```python
from build123d import *

# Parameters (mm, degrees)
BOSS_EXTRUDE1_DEPTH = 50.8
SKETCH3_R           = 1.27
CUT_EXTRUDE2_DEPTH  = 50.8
CUT_EXTRUDE1_DEPTH  = 50.8
CUT_EXTRUDE6_DEPTH  = 50.8
BOSS_EXTRUDE3_DEPTH = 20.32
SKETCH4_W           = 10.16
SKETCH4_H           = 15.24
CUT_EXTRUDE3_DEPTH  = 50.8
SKETCH5_R           = 2.54
CUT_EXTRUDE5_DEPTH  = 50.8
SKETCH8_R           = 2.54
BOSS_EXTRUDE2_DEPTH = 2.54
LPATTERN1_COUNT     = 2
LPATTERN1_PITCH     = 12.7
CUT_EXTRUDE7_DEPTH  = 20.32
SKETCH12_W          = 5.08
SKETCH12_H          = 19.941398178
CUT_EXTRUDE8_DEPTH  = 21.59
CUT_EXTRUDE9_DEPTH  = 5.08
LPATTERN2_COUNT     = 2
LPATTERN2_PITCH     = 15.24
CUT_EXTRUDE10_DEPTH = 40.767
BOSS_EXTRUDE4_START = 2.54
SKETCH16_R          = 7.638081415
BOSS_EXTRUDE4_DEPTH = 2.54
SKETCH17_R          = 2.54
CUT_EXTRUDE11_DEPTH = 2.54
SKETCH23_W          = 3.776239755
SKETCH23_H          = 7.410355269
CUT_EXTRUDE16_DEPTH = 2.54
CUT_EXTRUDE17_DEPTH = 9.906
SKETCH25_R          = 1.7526
CUT_EXTRUDE18_DEPTH = 20.828
SKETCH26_R          = 2.921
CUT_EXTRUDE19_DEPTH = 2.54


with BuildPart() as part:
    # Sketch1 → Boss-Extrude1 (new body)
    with BuildSketch(Plane(origin=(0, 0, 0), x_dir=(1, 0, 0), z_dir=(0, 1, 0))):
        with BuildLine():
            Line((-20.32, 27.095319289), (-20.32, 11.855319289))
            ThreePointArc((-20.32, 11.855319289), (-19.204076836, 9.161242453), (-16.51, 8.045319289))
            Line((-16.51, 8.045319289), (-3.81, 8.045319289))
            ThreePointArc((-3.81, 8.045319289), (-1.115923164, 9.161242453), (0, 11.855319289))
            Line((0, 11.855319289), (0, 27.095319289))
            ThreePointArc((0, 27.095319289), (-1.115923164, 29.789396126), (-3.81, 30.905319289))
            Line((-3.81, 30.905319289), (-16.51, 30.905319289))
            ThreePointArc((-16.51, 30.905319289), (-19.204076836, 29.789396126), (-20.32, 27.095319289))
        make_face()
    extrude(amount=BOSS_EXTRUDE1_DEPTH)

    # Sketch3 → Cut-Extrude2 (cut)
    with BuildSketch(Plane(origin=(0, 50.8, 0), x_dir=(1, 0, 0), z_dir=(0, 1, 0))):
        with Locations(Location((-10.16, 10.585319289, 0), (0, 0, 270))):
            Circle(SKETCH3_R)
        with Locations(Location((-10.16, 28.365319289, 0), (0, 0, 270))):
            Circle(SKETCH3_R)
    extrude(amount=-CUT_EXTRUDE2_DEPTH, mode=Mode.SUBTRACT)

    # Sketch2 → Cut-Extrude1 (cut)
    with BuildSketch(Plane.ZY.offset(20.32)):
        with BuildLine():
            Line((-27.095319289, 7.62), (-30.905319289, 15.24))
            Line((-30.905319289, 15.24), (-30.905319289, -5.08))
            Line((-30.905319289, -5.08), (-8.045319289, -5.08))
            Line((-8.045319289, -5.08), (-8.045319289, 15.24))
            Line((-8.045319289, 15.24), (-11.855319289, 7.62))
            ThreePointArc((-11.855319289, 7.62), (-19.475319289, 0), (-27.095319289, 7.62))
        make_face()
        with BuildLine():
            Line((-11.821559044, 42.970355269), (-8.045319289, 35.56))
            Line((-8.045319289, 35.56), (-8.045319289, 55.88))
            Line((-8.045319289, 55.88), (-30.905319289, 55.88))
            Line((-30.905319289, 55.88), (-30.905319289, 35.56))
            Line((-30.905319289, 35.56), (-27.092422036, 42.951560486))
            ThreePointArc((-27.092422036, 42.951560486), (-19.46663852, 50.799994215), (-11.821559044, 42.970355269))
        make_face()
    extrude(amount=-CUT_EXTRUDE1_DEPTH, mode=Mode.SUBTRACT)

    # Sketch7 → Cut-Extrude6 (cut)
    with BuildSketch(Plane.XY.offset(-8.045319289)):
        Polygon((-15.24, 50.8), (-12.7, 50.8), (-12.7, 35.56), (-7.62, 35.56), (-7.62, 50.8), (-5.08, 50.8), (-5.08, 35.56), (0, 35.56), (0, 59.156438057), (-20.32, 59.156438057), (-20.32, 35.56), (-15.24, 35.56), align=None)
    extrude(amount=-CUT_EXTRUDE6_DEPTH, mode=Mode.SUBTRACT)

    # Sketch9 → Boss-Extrude3 (add)
    with BuildSketch(Plane.ZY.offset(20.32)):
        with BuildLine():
            Line((-19.475319289, 35.56), (-30.961107471, 35.56))
            Line((-30.961107471, 35.56), (-30.961107471, 45.935432902))
            ThreePointArc((-30.961107471, 45.935432902), (-30.291229548, 47.014503778), (-29.026975399, 46.892882091))
            Line((-29.026975399, 46.892882091), (-27.092843326, 42.985764183))
            ThreePointArc((-27.092843326, 42.985764183), (-24.794356941, 37.723605727), (-19.475319289, 35.56))
        make_face()
    extrude(amount=-BOSS_EXTRUDE3_DEPTH)

    # Sketch4 → Cut-Extrude3 (cut)
    with BuildSketch(Plane.XY.offset(-8.045319289)):
        with Locations((-10.16, 7.62)):
            Rectangle(SKETCH4_W, SKETCH4_H)
    extrude(amount=-CUT_EXTRUDE3_DEPTH, mode=Mode.SUBTRACT)

    # Sketch5 → Cut-Extrude5 (cut)
    with BuildSketch(Plane.ZY.offset(20.32)):
        with Locations((-19.475319289, 7.62)):
            Circle(SKETCH5_R)
    extrude(amount=-CUT_EXTRUDE5_DEPTH, mode=Mode.SUBTRACT)

    # Sketch8 → Boss-Extrude2 (add)
    with BuildSketch(Plane.ZY.offset(15.24)):
        with Locations(Location((-19.441559044, 43.179995622, 0), (0, 0, 180))):
            Circle(SKETCH8_R)
    boss_extrude2 = extrude(amount=BOSS_EXTRUDE2_DEPTH)

    # LPattern1: Boss-Extrude2 ×2
    with Locations(*[(i * LPATTERN1_PITCH, 0, 0) for i in range(1, LPATTERN1_COUNT)]):
        add(boss_extrude2)

    # Sketch10 → Cut-Extrude7 (cut)
    with BuildSketch(Plane.XZ.offset(-35.56)):
        with BuildLine():
            Line((-16.51, -30.905319289), (-3.81, -30.905319289))
            ThreePointArc((-3.81, -30.905319289), (-1.115923164, -29.789396126), (0, -27.095319289))
            Line((0, -27.095319289), (5.770912039, -37.258829719))
            Line((5.770912039, -37.258829719), (-26.797758959, -37.890739908))
            Line((-26.797758959, -37.890739908), (-20.32, -27.095319289))
            ThreePointArc((-20.32, -27.095319289), (-19.204076836, -29.789396126), (-16.51, -30.905319289))
        make_face()
    extrude(amount=-CUT_EXTRUDE7_DEPTH, mode=Mode.SUBTRACT)

    # Sketch12 → Cut-Extrude8 (cut)
    with BuildSketch(Plane.XY.offset(-8.045319289)):
        with Locations((-10.16, 45.530699089)):
            Rectangle(SKETCH12_W, SKETCH12_H)
    extrude(amount=-CUT_EXTRUDE8_DEPTH, mode=Mode.SUBTRACT)

    # Sketch13 → Cut-Extrude9 (cut)
    with BuildSketch(Plane.ZY.offset(20.32)):
        Polygon((-19.475319289, 35.56), (-8.045319289, 30.82545932), (-1.320705488, 30.82545932), (-1.320705488, 35.56), align=None)
    cut_extrude9 = extrude(amount=-CUT_EXTRUDE9_DEPTH, mode=Mode.SUBTRACT)

    # LPattern2: Cut-Extrude9 ×2
    with Locations(*[(i * LPATTERN2_PITCH, 0, 0) for i in range(1, LPATTERN2_COUNT)]):
        add(cut_extrude9, mode=Mode.SUBTRACT)

    # Sketch15 → Cut-Extrude10 (cut, symmetric)
    with BuildSketch(Plane(origin=(0, 35.56, 0), x_dir=(1, 0, 0), z_dir=(0, 1, 0))):
        with BuildLine():
            Line((-10.16, 25.825319289), (-10.16, 13.125319289))
            ThreePointArc((-10.16, 13.125319289), (-7.62, 10.585319289), (-10.16, 8.045319289))
            Line((-10.16, 8.045319289), (-39.973745678, -4.467023153))
            Line((-39.973745678, -4.467023153), (-44.095820535, 43.963158694))
            Line((-44.095820535, 43.963158694), (-10.16, 30.905319289))
            ThreePointArc((-10.16, 30.905319289), (-12.7, 28.365319289), (-10.16, 25.825319289))
        make_face()
    extrude(amount=CUT_EXTRUDE10_DEPTH, both=True, mode=Mode.SUBTRACT)

    # Sketch16 → Boss-Extrude4 (add)
    with BuildSketch(Plane.ZY.offset(7.62).offset(BOSS_EXTRUDE4_START)):
        with Locations((-19.457237874, 43.161918585)):
            Circle(SKETCH16_R)
    extrude(amount=-BOSS_EXTRUDE4_DEPTH)

    # Sketch17 → Cut-Extrude11 (cut)
    with BuildSketch(Plane.ZY.offset(10.16)):
        with Locations((-19.457237874, 43.161918585)):
            Circle(SKETCH17_R)
    extrude(amount=-CUT_EXTRUDE11_DEPTH, mode=Mode.SUBTRACT)

    # Sketch23 → Cut-Extrude16 (cut)
    with BuildSketch(Plane(origin=(-5.08, 0, 0), x_dir=(0, 0, -1), z_dir=(1, 0, 0))):
        with Locations((9.933439167, 39.265177635)):
            Rectangle(SKETCH23_W, SKETCH23_H)
    extrude(amount=-CUT_EXTRUDE16_DEPTH, mode=Mode.SUBTRACT)

    # Sketch24 → Cut-Extrude17 (cut)
    with BuildSketch(Plane(origin=(-5.08, 0, 0), x_dir=(0, 0, -1), z_dir=(1, 0, 0))):
        Polygon((8.045319289, 35.56), (11.821559044, 35.56), (11.821559044, 32.38965536), (8.045319289, 30.82545932), align=None)
    extrude(amount=-CUT_EXTRUDE17_DEPTH, mode=Mode.SUBTRACT)

    # Sketch25 → Cut-Extrude18 (cut)
    with BuildSketch(Plane.ZY.offset(10.16)):
        with Locations((-19.475319289, 22.86)):
            Circle(SKETCH25_R)
    extrude(amount=-CUT_EXTRUDE18_DEPTH, mode=Mode.SUBTRACT)

    # Sketch26 → Cut-Extrude19 (cut)
    with BuildSketch(Plane(origin=(0, 0, 0), x_dir=(0, 0, -1), z_dir=(1, 0, 0))):
        with Locations((19.475319289, 22.86)):
            Circle(SKETCH26_R)
    extrude(amount=-CUT_EXTRUDE19_DEPTH, mode=Mode.SUBTRACT)


solid = part.part
```
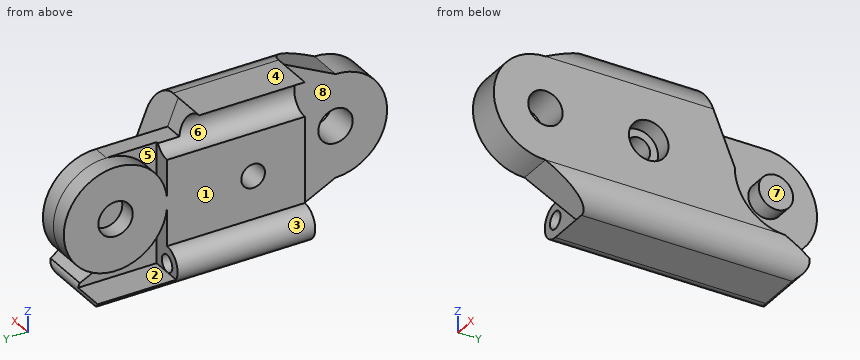
Build history of the part. All positions in model axes, mm. Face numbers are marked on the shaded views. A direction names the side the tool comes from. Coordinates: 2 decimals unless noted, no trailing zeros. Write each loop counter-clockwise with the first axis right and the second up, starting at its lowest first coordinate (ties: lowest second). Pieces come first, ordered by that corner, then holes.
1. Band-saw the part on A-A, the plane y = 22.86. Give the cut face in (x, z), and give its area (3 significant figures).
Answer block:
outline: (-10.16, -30.91) - (-3.81, -30.91) arc R3.81 ccw to (0, -27.1) - (0, -22.4) - (-2.54, -22.4) - (-2.54, -21.23) - (-10.16, -21.23) - (-10.16, -25.83) arc R2.54 ccw to start; (-10.16, -17.72) - (-2.54, -17.72) - (-2.54, -16.55) - (0, -16.55) - (0, -11.86) arc R3.81 ccw to (-3.81, -8.05) - (-10.16, -8.05) arc R2.54 cw to (-10.16, -13.13) - close; hole circle Ø2.54 at (-10.16, -28.37)
area: 179 mm2
2. Drill centre lines: probe 1 along Y at (x, z) = (-4, -21.5); probe 2 along X at (y, z) = (24.5, -16.5); probe 3 along X at (y, z) = (41, -17.5). Where is each one in solid material? Low to high.
Answer block:
probe 1: y = 0.27 to 6.09, 9.15 to 35.83, 41.69 to 44.67
probe 2: x = -10.16 to 0
probe 3: x = -10.16 to -5.08
3. Drop flat-ended pins along their axis: pin 1 (7.5 mm diameter, centred on y = 44, z = -26, fed in from -X); pin 2 (3 mm diameter, centred on x = -7, z = -25.5, fed in from -Y); pin 3 (4 mm diameter, centred on y = 43.16, z = -19.46, fed in from -X). Give the stop position or say it passes through.
Answer block:
pin 1: stops at x = -12.36
pin 2: stops at y = 15.24
pin 3: stops at x = -7.62
4. Band-saw the part on D-D, the plane z = -23. Give the cut face in (x, y), and give its area (3 significant figures).
Answer block:
outline: (-10.16, 15.24) - (-5.08, 15.24) - (-5.08, 0.86) - (0, 0.86) - (0, 36.42) - (-5.08, 36.42) - (-5.08, 49.93) - (-10.16, 49.93) - (-10.16, 36.4) - (-7.62, 36.4) - (-7.62, 35.56) - (-10.16, 35.56) - close
area: 355 mm2
5. Band-saw the part on B-B, the plane x = -6.75. Give the cut face in (y, z).
Answer block:
outline: (15.24, -30.91) - (46.3, -30.91) arc R1.2 ccw to (46.89, -29.03) - (42.99, -27.09) arc R7.64 ccw (long way) to (42.97, -11.82) - (32.39, -11.82) - (30.83, -8.05) - (15.24, -8.05) - close; hole circle Ø3.51 at (22.86, -19.48)
6. Pull direction Z, two halves, no side cores. Call the marked faces 1, 2, 3 and 4: released by +Z, released by -Z, zero draft, split by the parting line, or undercut.
Answer block:
face 1: zero draft
face 2: undercut
face 3: split by the parting line
face 4: released by +Z
7. Band-saw the part on C-C, the plane y = 16. Give the cut face in (x, z).
Answer block:
outline: (-10.16, -30.91) - (-3.81, -30.91) arc R3.81 ccw to (0, -27.1) - (0, -11.86) arc R3.81 ccw to (-3.81, -8.05) - (-10.16, -8.05) arc R2.54 cw to (-10.16, -13.13) - (-10.16, -25.83) arc R2.54 ccw to start; hole circle Ø2.54 at (-10.16, -28.37)
8. 3-axis set-ups, long thin cutter, end or side, ignore diameter. For the marked faces 5, 6, 7 and 8: which of +Z, -Z, +X, -X, +Y, -Y reach the whole face in a straight line?
Answer block:
face 5: +Z, -X
face 6: -X, -Y
face 7: +Z, +X, +Y
face 8: +Z, -Z, -X, -Y
